Work out the finished part from the listing and answer in its coordinate system (mm). A direction names the side the tool comes from. Give positions to 0.01 mm unless a question says otherwise; leave off trailing zeros. Write each loop counter-clockwise with the first axis right and the second up, starting at its lowest first coordinate (ties: lowest second). Pieces come first, ordered by that corner, then holes. Notation, with made-up numbers: (-38.75, 67.25) - (11.25, 67.25) arc R19 cw to (11.25, 82.25) - close; hole circle Ø11 at (28, 14.5). An arc over 180 degrees is marked (long way). Write item = value, one per line.
from build123d import *

# Parameters (mm, degrees)
F0_W     = 380
F0_H     = 140
F1_DEPTH = 32
F2_T     = -2.5
F3_DEPTH = 2.5
F4_DEPTH = 2.5
F5_W     = 8
F5_H     = 60
F6_DEPTH = 2.5


with BuildPart() as f1:
    # F0 (on Right) → F1 (new body)
    with BuildSketch(Plane.YZ):
        Rectangle(F0_W, F0_H)
    extrude(amount=F1_DEPTH)

    # F2
    f2_openings = [f1.faces().sort_by_distance(p)[0] for p in [
        (16, -190, 0),
    ]]
    offset(amount=F2_T, openings=f2_openings)

    # F3 (cut): a face of the model
    f3_faces = [f1.faces().sort_by_distance(p)[0] for p in [
        (16, 0, -70),
    ]]
    extrude(f3_faces, amount=-F3_DEPTH, mode=Mode.SUBTRACT)

    # F4 (cut): a face of the model
    f4_faces = [f1.faces().sort_by_distance(p)[0] for p in [
        (16, 190, 1.25),
    ]]
    extrude(f4_faces, amount=-F4_DEPTH, mode=Mode.SUBTRACT)

    # F5 (on face) → F6 (cut, through all)
    with BuildSketch(Plane.YZ.offset(32)):
        with Locations((-164.3113616109, -34.5)):
            Rectangle(F5_W, F5_H)
        with Locations((-115.6886383891, -34.5)):
            Rectangle(F5_W, F5_H)
        with Locations((24.3113616109, -34.5)):
            Rectangle(F5_W, F5_H)
        with Locations((-24.3113616109, -34.5)):
            Rectangle(F5_W, F5_H)
        with Locations((164.3113616109, -34.5)):
            Rectangle(F5_W, F5_H)
        with Locations((115.6886383891, -34.5)):
            Rectangle(F5_W, F5_H)
    extrude(amount=-F6_DEPTH, mode=Mode.SUBTRACT)


solid = f1.part
1. For a pull along X with two mould halves and no side action, classify faces 3 (the flat face through (32, -4, 2)), 4 (the flat face through (16, -4, 67.5)), 5 (the flat face through (2, 187.5, 1)) as pulls with the +X half, pulls with the -X half, needs draft (parallel to the pull), parting line crosses it, or undercut.
Solution:
face_3 = pulls with the +X half
face_4 = undercut
face_5 = needs draft
2. Find section B-B, the plane z = -17. Give the number of separate pieces and of enclosed holes in the cut face, then the cut area to 3 significant figures.
Solution:
separate_pieces = 8
enclosed_holes = 0
area = 1,770 mm^2
3. A tool of negligible diameter and unlimited length cuts with its end or side. For faces 1 (the flat face through (2.5, -4, 1)), 2 (the flat face through (2, -190, 1)), from which of +Z, -Z, +X, -X, +Y, -Y can it reach the whole face along a straight path? Write none if from no direction.
Solution:
face_1 = -Z, +Y, -Y
face_2 = +Z, -Z, +X, -X, -Y
4. Straight lines are drawn through the part: line 1 (X direction, y = 105, z = 38.5); line 2 (Z direction, x = 3, y = 69). For each, find the intervals that lie inside material, in ascending order.
Solution:
line_1 = 0 to 2.5, 29.5 to 32
line_2 = 67.5 to 70
5. Find section A-A, the plane z = 48. Give the vertices of the cut face in (x, y).
Solution:
outline = (0, -190) - (2.5, -190) - (2.5, 187.5) - (0, 187.5) - close; (29.5, -190) - (32, -190) - (32, 187.5) - (29.5, 187.5) - close
6. Find section C-C, the plane y = 145. Give the vertices of the cut face in (x, z).
Solution:
outline = (0, -67.5) - (2.5, -67.5) - (2.5, 67.5) - (29.5, 67.5) - (29.5, -67.5) - (32, -67.5) - (32, 70) - (0, 70) - close
7. Find section D-D, the plane x = 9. Give the vertices of the cut face in (y, z).
Solution:
outline = (-190, 67.5) - (187.5, 67.5) - (187.5, 70) - (-190, 70) - close
8. Given pin 1 (2 mm diameter, centred on x = 5, y = 133, fed in from -Z), flat-ended and moving along its own axis, determine where the tip first touches the part or whether it passes through.
Solution:
pin_1 = 67.5
